Source: CAD feature listing. Evaluate the final solid. Frame: model axes, mm. Round coordinates to 2 decimals unless told otherwise and drop trailing zeros. Loops run counter-clockwise (first coordinate to the right, second up) from the corner with the lowest first, then second, coordinate; pieces in that order, holes last.
(1) Section B-B, the plane x = -5. Return the cut outline in (y, z).
(2) Material intervals for probe 1 along Z at (x, y) = (6.5, -3.5), sorted ascending.
(3) Section C-C, the plane y = -5. Return the cut outline in (x, z), plus the area to 3 significant figures.
(4) Section A-A, the plane z = 26.75. Return the cut outline in (x, y).
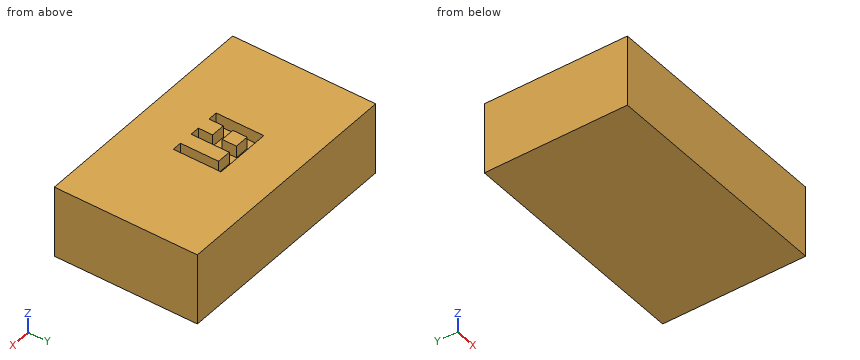
Autodesk Fusion 360 part; units mm, degrees
sketch "Skizze1" plane through (0, 0, 0) normal (0, 0, 1) x (1, 0, 0)
  line L0 (50, -30) -> (-50, -30)
  line L1 (-50, -30) -> (-50, 30)
  line L2 (-50, 30) -> (50, 30)
  line L3 (50, 30) -> (50, -30)
  line L4 (50, -30) -> (-50, 30) construction
  line L5 (-50, -30) -> (50, 30) construction
  dimension "d1" = 100
  dimension "d2" = 60
extrude "Extrusion1" add sketch "Skizze1" along normal blind 30
sketch "Skizze2" plane through (0, 0, 30) normal (0, 0, 1) x (-1, 0, 0)
  line L0 (-50, -30) -> (50, -30)
  line L1 (50, -30) -> (50, 30)
  line L2 (50, 30) -> (-50, 30)
  line L3 (-50, 30) -> (-50, -30)
  line L4 (10, 10) -> (14, 10)
  line L5 (14, 10) -> (14, -10)
  line L6 (14, -10) -> (10, -10)
  line L7 (0, -6) -> (0, 10)
  line L8 (4, -10) -> (0, -10)
  line L9 (0, 10) -> (4, 10)
  line L10 (-6, 10) -> (-6, -6)
  line L11 (-10, -10) -> (-10, 10)
  line L12 (-6, -10) -> (-10, -10)
  line L13 (-10, 10) -> (-6, 10)
  line L14 (14, -10) -> (-10, -10)
  line L15 (14, -10) -> (14, -6)
  line L16 (10, 0) -> (4, 0)
  line L17 (14, 0) -> (14, 4)
  line L18 (10, 4) -> (4, 4)
  line L19 (10, -6) -> (10, 0)
  line L20 (10, 4) -> (10, 10)
  line L21 (4, 10) -> (4, 4)
  line L22 (4, 0) -> (4, -6)
  line L23 (10, -6) -> (4, -6)
  line L24 (0, -6) -> (-6, -6)
  dimension "d5" = 4
  dimension "d10" = 4
  dimension "d11" = 4
extrude "Extrusion2" cut sketch "Skizze2" against normal blind 5 contours L4 L5 L6 L7 L8 L9 L10 L11 L12 L13 L14 L15 L17 L18 L20 L21 L24
Output values:
1. outline: (-30, 0) - (30, 0) - (30, 30) - (10, 30) - (10, 25) - (6, 25) - (6, 30) - (0, 30) - (0, 25) - (-4, 25) - (-4, 30) - (-30, 30) - close
2. probe 1: z = 0 to 25
3. outline: (-50, 0) - (50, 0) - (50, 30) - (10, 30) - (10, 25) - (6, 25) - (6, 30) - (0, 30) - (0, 25) - (-4, 25) - (-4, 30) - (-10, 30) - (-10, 25) - (-14, 25) - (-14, 30) - (-50, 30) - close
3. area: 2,940 mm2
4. outline: (-50, -30) - (50, -30) - (50, 30) - (-50, 30) - close; (-10, 0) - (-4, 0) - (-4, 6) - (-10, 6) - close; hole (-14, -10) - (-10, -10) - (-10, -4) - (-4, -4) - (-4, -10) - (0, -10) - (0, 6) - (6, 6) - (6, -10) - (10, -10) - (10, 10) - (-14, 10) - close
